Input: part model. Units: mm. Frame: model coordinates. Give positions to 0.01 mm unless a question says otherwise; leave off trailing zeros. Loops run counter-clockwise (first coordinate to the right, second up) from the corner with the lowest first, then second, coordinate; pieces in that order, holes last. Notation, with made-up numbers: (48, -10.5) -> (64, -10.5) arc R17 cw to (64, -6.5) -> close; hole circle Ø1 at (80.5, 15.5). An arc over 180 degrees is marked (long way). Answer as a JSON object with one key per item and string values.
```python
from build123d import *

# Parameters (mm, degrees)
F0_W     = 200
F0_H     = 90
F0_R     = 29.6278920172
F1_DEPTH = 38.1
F2_DEPTH = 25.4


# Not quite as in the source:
# - a feature names something its author has since deleted; it is built from what else it names


with BuildPart() as f1:
    # F0 (on Front) → F1 (new body)
    with BuildSketch(Plane.XZ):
        Rectangle(F0_W, F0_H)
        Circle(F0_R, mode=Mode.SUBTRACT)
    extrude(amount=F1_DEPTH)

    # F2 (cut): a face of the model
    f2_faces = [f1.faces().sort_by_distance(p)[0] for p in [
        (0, -38.1, -42.8068287801),
    ]]
    extrude(f2_faces, amount=-F2_DEPTH, mode=Mode.SUBTRACT)


solid = f1.part
```
Q1. Section A-A, the plane x = 0. Return the cut outline in (y, z).
Evaluation:
{"outline": "(-12.7, -45) -> (0, -45) -> (0, -29.63) -> (-12.7, -29.63) -> close; (-12.7, 29.63) -> (0, 29.63) -> (0, 45) -> (-12.7, 45) -> close"}
Q2. Section B-B, the plane z = 0. Return the cut outline in (x, y), then the cut area to 3 significant figures.
Evaluation:
{"outline": "(-100, -12.7) -> (-29.63, -12.7) -> (-29.63, 0) -> (-100, 0) -> close; (29.63, -12.7) -> (100, -12.7) -> (100, 0) -> (29.63, 0) -> close", "area": "1,790 mm2"}
Q3. Ray query, line 1 along Z through (x, y) = (0, -3); line 2 along X through (y, z) = (-6.5, -9.5); line 3 along X through (y, z) = (-4.75, 15). Return the intervals inside material, ascending.
Evaluation:
{"line 1": "z = -45 to -29.63, 29.63 to 45", "line 2": "x = -100 to -28.06, 28.06 to 100", "line 3": "x = -100 to -25.55, 25.55 to 100"}
Q4. Section C-C, the plane y = -8.5. Return the cut outline in (x, z), then the cut area to 3 significant figures.
Evaluation:
{"outline": "(-100, -45) -> (100, -45) -> (100, 45) -> (-100, 45) -> close; hole circle Ø59.26 at (0, 0)", "area": "15,200 mm2"}
Q5. Pin query (flat end, axial travel): pin 1 (1 mm diameter, centred on x = 27.5, z = 5, fed in from +Y). Return the tip coordinate at first contact, or that it passes through.
Evaluation:
{"pin 1": "passes through"}
Q6. Draft query along Z for faces 1 (the flat face through (-100, -6, -1)), 2 (the flat face through (-1, -6, 45)), 3 (the cylindrical face through (-6.423, -6.261, -28.923)). Return one class per face: +Z half, -Z half, draft (parallel to the pull), parting line (faces both ways), or undercut.
Evaluation:
{"face 1": "draft", "face 2": "+Z half", "face 3": "undercut"}
